Autodesk Inventor part; units mm, degrees
ref_plane "YZ Plane" through (0, 0, 0) normal (1, 0, 0) x (0, 1, 0)
ref_plane "XZ Plane" through (0, 0, 0) normal (0, 1, 0) x (-1, 0, 0)
ref_plane "XY Plane" through (0, 0, 0) normal (0, 0, 1) x (1, 0, 0)
sketch "Sketch3" plane through (0, 0, 0) normal (0, 0, 1) x (1, 0, 0)
  line L0 (-20.1, 21) -> (20.1, 21)
  line L1 (20.1, 21) -> (20.1, -21)
  line L2 (20.1, -21) -> (-20.1, -21)
  line L3 (-20.1, -21) -> (-20.1, 21)
  line L4 (-20.1, 21) -> (20.1, -21) construction
  line L5 (20.1, 21) -> (-20.1, -21) construction
  point P0 (0, 0)
  dimension "d24" = 40.2
  dimension "d25" = 42
extrude "Extrusion3" add sketch "Sketch3" along normal blind 1.5
sketch "Sketch4" plane through (0, 0, 1.5) normal (0, 0, 1) x (1, 0, 0)
  line L0 (20.1, 21) -> (-20.1, 21)
  line L1 (-20.1, 21) -> (-17.1, 21) construction
  line L2 (-17.1, 21) -> (-17.1, 18) construction
  line L3 (-17.1, 18) -> (-20.1, 18) construction
  line L4 (-20.1, 18) -> (-20.1, 21) construction
  circle A0 centre (-17.1, 18) radius 1.7
  point P0 (0, 0)
  dimension "d28" = 3
  dimension "d29" = 3
  dimension "d30" = 3.4
extrude "Extrusion4" cut sketch "Sketch4" against normal through all
fillet "Fillet2" radius 3 1 edges at (-20.1, 21, 0.75)
mirror "Mirror2" about plane through (0, 0, 0) normal (0, 1, 0) of "Fillet2", "Extrusion4"
mirror "Mirror3" about plane through (0, 0, 0) normal (1, 0, 0) of "Fillet2", "Extrusion4", "Mirror2"
sketch "Sketch5" plane through (0, 0, 1.5) normal (0, 0, 1) x (1, 0, 0)
  circle A0 centre (-17.1, 18) radius 1.7 construction
  circle A1 centre (17.1, 18) radius 1.7 construction
  line L0 (-17.1, 18) -> (17.1, 18) construction
  line L1 (17.1, 18) -> (17.1, 15) construction
  line L2 (17.1, 15) -> (-17.1, 15) construction
  line L3 (-17.1, 15) -> (-17.1, 18) construction
  arc A2 (-17.1, 21) -> (-20.1, 18) centre (-17.1, 18) ccw
  line L4 (-17.1, 18) -> (-17.1, 21) construction
  line L5 (17.1, 21) -> (-17.1, 21) construction
  line L6 (17.1, 18) -> (17.1, 21) construction
  arc A3 (20.1, 18) -> (17.1, 21) centre (17.1, 18) ccw construction
  line L7 (17.1, 21) -> (-17.1, 21) construction
  line L8 (-17.1, 18) -> (-17.1, 21) construction
  line L9 (-17.1, 21) -> (-16, 21) construction
  line L10 (-16, 21) -> (-16, 18) construction
  line L11 (-16, 18) -> (-17.1, 18) construction
  line L12 (17.1, 18) -> (17.1, 21) construction
  line L13 (17.1, 21) -> (16, 21) construction
  line L14 (16, 21) -> (16, 18) construction
  line L15 (16, 18) -> (17.1, 18) construction
  arc A4 (-16, 21) -> (16, 21) centre (0, 39.3333) ccw
  line L16 (-16, 21) -> (16, 21)
  point P0 (0, 0)
  point P1 (0, 15)
  dimension "d34" = 3
  dimension "d42" = 1.1
  dimension "d43" = 1.1
extrude "Extrusion5" cut sketch "Sketch5" against normal through all
mirror "Mirror4" about plane through (0, 0, 0) normal (0, 1, 0) of "Extrusion5"
fillet "Fillet3" radius 3 4 edges at (-16, 21, 0.75) (16, 21, 0.75) (16, -21, 0.75) (-16, -21, 0.75)
sketch "Sketch7" plane through (0, 0, 1.5) normal (0, 0, 1) x (1, 0, 0)
  line L0 (15.3, 7.9) -> (15.3, -11.6) construction
  line L1 (15.3, -11.6) -> (-15.4, -11.6) construction
  line L2 (-15.4, -11.6) -> (-15.4, 7.9) construction
  line L3 (-15.4, 7.9) -> (15.3, 7.9) construction
  line L4 (-17.65, -15) -> (30.6, -15) construction
  line L5 (30.6, -15) -> (30.6, 15) construction
  line L6 (30.6, 15) -> (-30.1, 15) construction
  line L7 (-30.1, 15) -> (-30.1, 10) construction
  line L8 (-17.65, 10) -> (-30.1, 10) construction
  line L9 (-17.65, 10) -> (-17.65, -15) construction
  line L10 (15.3, -11.6) -> (-15.4, 7.9) construction
  line L11 (-15.4, -11.6) -> (15.3, 7.9) construction
  line L12 (0, 0) -> (-0.05, 0) construction
  line L13 (-0.05, 0) -> (-0.05, -1.85) construction
  line L14 (-0.05, -1.85) -> (0, -1.85) construction
  line L15 (0, -1.85) -> (0, 0) construction
  circle A0 centre (0, -1.85) radius 9
  dimension "d41" = 18
extrude "Extrusion6" cut sketch "Sketch7" against normal through all
sketch "Sketch8" plane through (0, 0, 1.5) normal (0, 0, 1) x (1, 0, 0)
  circle A0 centre (0, -1.85) radius 9
  arc A1 (-17.088, -21) -> (-15.2125, -20.3415) centre (-17.088, -18) ccw
  arc A2 (15.2125, -20.3415) -> (-15.2125, -20.3415) centre (0, -39.3333) ccw
  arc A3 (15.2125, -20.3415) -> (17.088, -21) centre (17.088, -18) ccw
  line L0 (17.088, -21) -> (17.1, -21)
  arc A4 (17.1, -21) -> (20.1, -18) centre (17.1, -18) ccw
  line L1 (20.1, -18) -> (20.1, 18)
  arc A5 (20.1, 18) -> (17.1, 21) centre (17.1, 18) ccw
  line L2 (17.1, 21) -> (17.088, 21)
  arc A6 (17.088, 21) -> (15.2125, 20.3415) centre (17.088, 18) ccw
  arc A7 (-15.2125, 20.3415) -> (15.2125, 20.3415) centre (0, 39.3333) ccw
  arc A8 (-15.2125, 20.3415) -> (-17.088, 21) centre (-17.088, 18) ccw
  line L3 (-17.088, 21) -> (-17.1, 21)
  arc A9 (-17.1, 21) -> (-20.1, 18) centre (-17.1, 18) ccw
  line L4 (-20.1, 18) -> (-20.1, -18)
  arc A10 (-20.1, -18) -> (-17.1, -21) centre (-17.1, -18) ccw
  line L5 (-17.1, -21) -> (-17.088, -21)
  circle A11 centre (17.1, -18) radius 1.7
  circle A12 centre (17.1, 18) radius 1.7
  circle A13 centre (-17.1, -18) radius 1.7
  circle A14 centre (-17.1, 18) radius 1.7
  line L6 (21.1, 18) -> (21.1, -18)
  arc A15 (17.1, -22) -> (21.1, -18) centre (17.1, -18) ccw
  line L7 (17.1, -22) -> (17.088, -22)
  arc A16 (14.5873, -21.122) -> (17.088, -22) centre (17.088, -18) ccw
  arc A17 (14.5873, -21.122) -> (-14.5873, -21.122) centre (0, -39.3333) ccw
  arc A18 (-17.088, -22) -> (-14.5873, -21.122) centre (-17.088, -18) ccw
  line L8 (-17.088, -22) -> (-17.1, -22)
  arc A19 (-21.1, -18) -> (-17.1, -22) centre (-17.1, -18) ccw
  line L9 (-21.1, -18) -> (-21.1, 18)
  arc A20 (-17.1, 22) -> (-21.1, 18) centre (-17.1, 18) ccw
  line L10 (-17.1, 22) -> (-17.088, 22)
  arc A21 (-14.5873, 21.122) -> (-17.088, 22) centre (-17.088, 18) ccw
  arc A22 (-14.5873, 21.122) -> (14.5873, 21.122) centre (0, 39.3333) ccw
  arc A23 (17.088, 22) -> (14.5873, 21.122) centre (17.088, 18) ccw
  line L11 (17.088, 22) -> (17.1, 22)
  arc A24 (21.1, 18) -> (17.1, 22) centre (17.1, 18) ccw
  point P0 (0, 0)
  dimension "d44" = 1
extrude "Extrusion7" add sketch "Sketch8" against normal up to surface (1.5 mm away) contours L6 A15 L7 A16 A17 A18 L8 A19 L9 A20 L10 A21 A22 A23 L11 A24
equation "\"d43\" = d42"
properties part number "seal"
Here's how the part is built. I have some questions about the finished solid (model axes, mm). A direction names the side the tool comes from. Coordinates: 2 decimals unless noted, no trailing zeros. Order: outer loops, then holes, each group sorted by start corner. A loop starts at its lowest first (then second) coordinate and runs counter-clockwise, first axis right, second up. Notation, with made-up numbers: M 71,72.5 L 101,72.5 A25 cw 101,97.5 Z; hole C -21.75,30.5 d4. An arc over 180 degrees is marked long. Answer as a JSON object with one key per item and string values. Group by question number.
(1) Suppose I cut it at D-D, the plane y = 17.5. Please give me the cut outline in (x, z), then the cut area to 3 significant figures.
(2) Suppose I cut it at A-A, the plane x = 0. Please give me the cut outline in (y, z).
(3) I need wall thicknesses on probe 1 along Y at (x, z) = (-17, 0.3); probe 2 along X at (y, z) = (19, 1); probe 3 along Y at (x, z) = (-16.5, 1.35). Which ranges of each line are inside material? Lowest first, please.
(4) For pin 1 (2 mm diameter, centred on x = -17.1, y = -18, fed in from +Z), with a flat end and sliding along its axis, tell me the tip position at first contact or that it passes through.
(5) Suppose I cut it at C-C, the plane z = 1.05. State how many separate pieces and enclosed holes the cut face has, then the cut area to 3 significant figures.
(6) If we mould it in two halves opening along Y, with no side actions, what happens to faces 1 (the face through (19.897, -20.859, 0.76)), 2 (the face through (-8.99, -1.45, 0.76)), 3 (the face through (-15.745, 21.768, 0.76)), 4 (the face through (-10, 0, 1.5))? For each: released by +Y, released by -Y, zero draft, split by the parting line, or undercut.
(7) Which directions (+Z, -Z, +X, -X, +Y, -Y) give clear straight access to the entire face, cutting with the end or side of a thin tool? Please do faces 5 (the face through (15.78, 21.78, 0.76)), 6 (the face through (15.745, -21.768, 0.76)), 7 (the face through (-19.897, 20.859, 0.76)).
(8) Suppose I cut it at B-B, the plane y = -10. Please give me the cut outline in (x, z), then the cut area to 3 significant figures.
Values found:
{
 "1": {"outline": "M -21.1,0 L -18.72,0 L -18.72,1.5 L -21.1,1.5 Z; M -15.48,0 L -8.23,0 L -8.23,1.5 L -15.48,1.5 Z; M 8.23,0 L 15.48,0 L 15.48,1.5 L 8.23,1.5 Z; M 18.72,0 L 21.1,0 L 21.1,1.5 L 18.72,1.5 Z", "area": "28.9 mm^2"},
 "2": {"outline": "M -16,0 L -10.85,0 L -10.85,1.5 L -16,1.5 Z; M 7.15,0 L 16,0 L 16,1.5 L 7.15,1.5 Z"},
 "3": {"probe 1": "y = -22 to -19.7, -16.3 to 16.3, 19.7 to 22", "probe 2": "x = -20.97 to -18.47, -15.73 to -11.45, 11.45 to 15.73, 18.47 to 20.97", "probe 3": "y = -21.96 to -19.59, -16.41 to 16.41, 19.59 to 21.96"},
 "4": {"pin 1": "passes through"},
 "5": {"separate pieces": "1", "enclosed holes": "5", "area": "1,290 mm^2"},
 "6": {"face 1": "released by -Y", "face 2": "undercut", "face 3": "released by +Y", "face 4": "zero draft"},
 "7": {"face 5": "+Z, -Z, +Y", "face 6": "+Z, -Z, -Y", "face 7": "+Z, -Z, -X, +Y"},
 "8": {"outline": "M -21.1,0 L -3.82,0 L -3.82,1.5 L -21.1,1.5 Z; M 3.82,0 L 21.1,0 L 21.1,1.5 L 3.82,1.5 Z", "area": "51.8 mm^2"}
}
